Design review of the part shown in the three views and the two pictorial views. Dimensions are in mm from the part's minimum x, y and z. Coordinates: 2 decimals unless noted, no trailing zeros. Order: outer loops, then holes, each group sorted by start corner. A loop starts at its lowest first (then second) coordinate and runs counter-clockwise, first axis right, second up. Notation, with made-up numbers: (-30.75, 74.5) -> (5.25, 74.5) arc R14 ccw to (5.25, 89.5) -> close; hole circle Ø11 at (-7.5, 41.5). An arc over 180 degrees is marked (long way). Answer as a JSON object with one key per item and string values. Group by question number.
1) Add section D-D, the plane x = 17.5. Write out the cut boundary in (y, z).
2) Wall thickness on L1, parallel to X at y = 0.3, z = 17.75 (1 decimal); L2, parallel to X at y = 0.1, z = 18 (1 decimal); L3, parallel to Z at x = 9.75, y = 0.15: over which ranges is each line inside the solid? List them lowest first.
3) Add section C-C, the plane z = 1. Write out the cut boundary in (x, y).
4) Add section B-B, the plane x = 14.25. Write out the cut boundary in (y, z) (1 decimal).
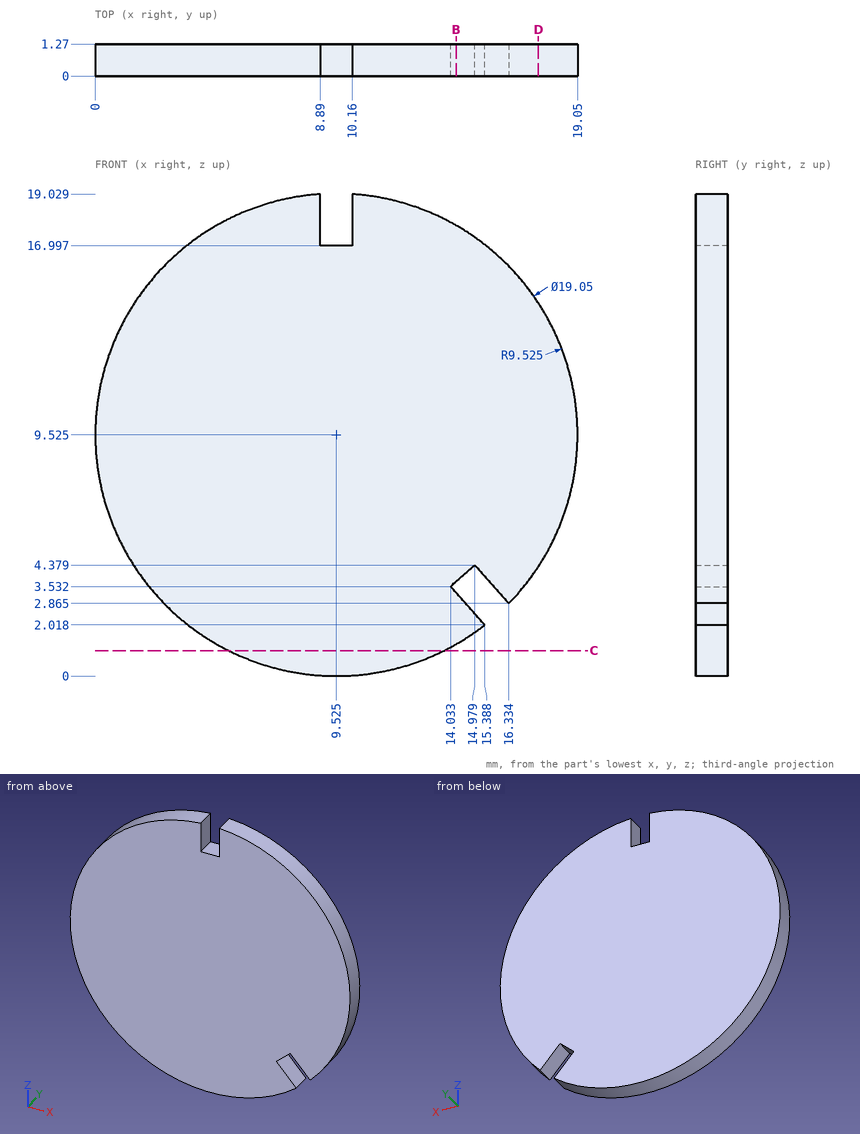
Output values:
{
 "1": {"outline": "(0, 4.32) -> (1.27, 4.32) -> (1.27, 14.73) -> (0, 14.73) -> close"},
 "2": {"L1": "x = 4.7 to 8.9, 10.2 to 14.3", "L2": "x = 5.2 to 8.9, 10.2 to 13.9", "L3": "z = 0 to 17"},
 "3": {"outline": "(5.28, 0) -> (13.77, 0) -> (13.77, 1.27) -> (5.28, 1.27) -> close"},
 "4": {"outline": "(0, 1.3) -> (1.3, 1.3) -> (1.3, 3.3) -> (0, 3.3) -> close; (0, 3.7) -> (1.3, 3.7) -> (1.3, 17.8) -> (0, 17.8) -> close"}
}
